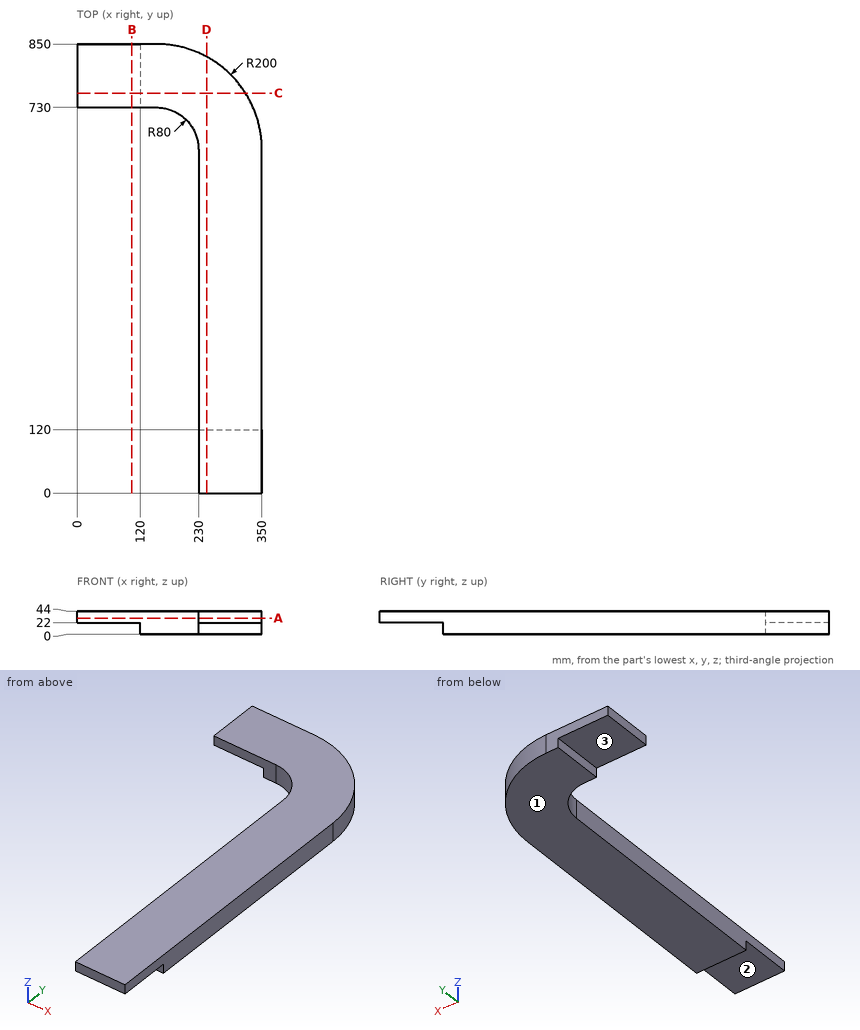
Could you check a few things on this drawing? It's one solid part, dimensions in mm from its lowest x, y, z. A direction names the side the tool comes from. Coordinates: 2 decimals unless noted, no trailing zeros. Order: outer loops, then holes, each group sorted by start corner. A loop starts at its lowest first (then second) coordinate and runs counter-clockwise, first axis right, second up. Notation, with made-up numbers: (18.25, -12) - (47.25, -12) arc R20 ccw to (47.25, -6) - close; hole circle Ø8 at (71, 54.5). An arc over 180 degrees is marked (long way). Answer as a JSON object with one key per item and string values. Group by question number.
Q1. I need wall thicknesses on line 1 (X direction, y = 465, z = 6); line 2 (Y direction, x = 149, z = 21); line 3 (X direction, y = 808, z = 22.5). Which ranges of each line are inside material? Lowest first, please. Write a range as from..to.
Q2. Imagine slicing it at C-C (y = 757). Please give me the cut outline in (x, z), and give its area (3 significant figures).
Q3. Imagine slicing it at D-D (x = 245.5). Please give me the cut outline in (y, z), and give its area (3 significant figures).
Q4. Will these pins go through, and if not, where does the flat tip stop? P1, Ø17.5, axis at x = 295, z = 12, coming from the -Y side; P2, Ø6, axis at x = 233.5, y = 754.5, coming from the -Z side; P3, Ø4, axis at y = 533.5, z = 6.5, coming from the -X side; P4, Ø24, axis at y = 810.5, z = 9, coming from the -X side.
Q5. Imagine slicing it at A-A (z = 30.5). Please give me the cut outline in (x, y), and give its area (3 significant figures).
Q6. On a 3-axis mill with a long thin cutter (end or side, diameter ignored), from which of +Z, -Z, +X, -X, +Y, -Y can I reach the whole of each face in a straight line? I mean the marked faces 1, 2 and 3. Say none if no direction works.
Q7. Imagine slicing it at B-B (x = 104). Please give me the cut outline in (y, z).
Determined:
{
 "1": {"line 1": "x = 230..350", "line 2": "y = 730..850", "line 3": "x = 0..272.62"},
 "2": {"outline": "(0, 22) - (120, 22) - (120, 0) - (318.97, 0) - (318.97, 44) - (0, 44) - close", "area": "11,400 mm2"},
 "3": {"outline": "(0, 22) - (120, 22) - (120, 0) - (825.73, 0) - (825.73, 44) - (0, 44) - close", "area": "33,700 mm2"},
 "4": {"P1": "stops at y = 120", "P2": "stops at z = 0", "P3": "stops at x = 230", "P4": "stops at x = 120"},
 "5": {"outline": "(0, 730) - (150, 730) arc R80 cw to (230, 650) - (230, 0) - (350, 0) - (350, 650) arc R200 ccw to (150, 850) - (0, 850) - close", "area": "122,000 mm2"},
 "6": {"face 1": "-Z, +X, -X, +Y, -Y", "face 2": "-Z, +X, -X, -Y", "face 3": "-Z, -X, +Y, -Y"},
 "7": {"outline": "(730, 22) - (850, 22) - (850, 44) - (730, 44) - close"}
}
